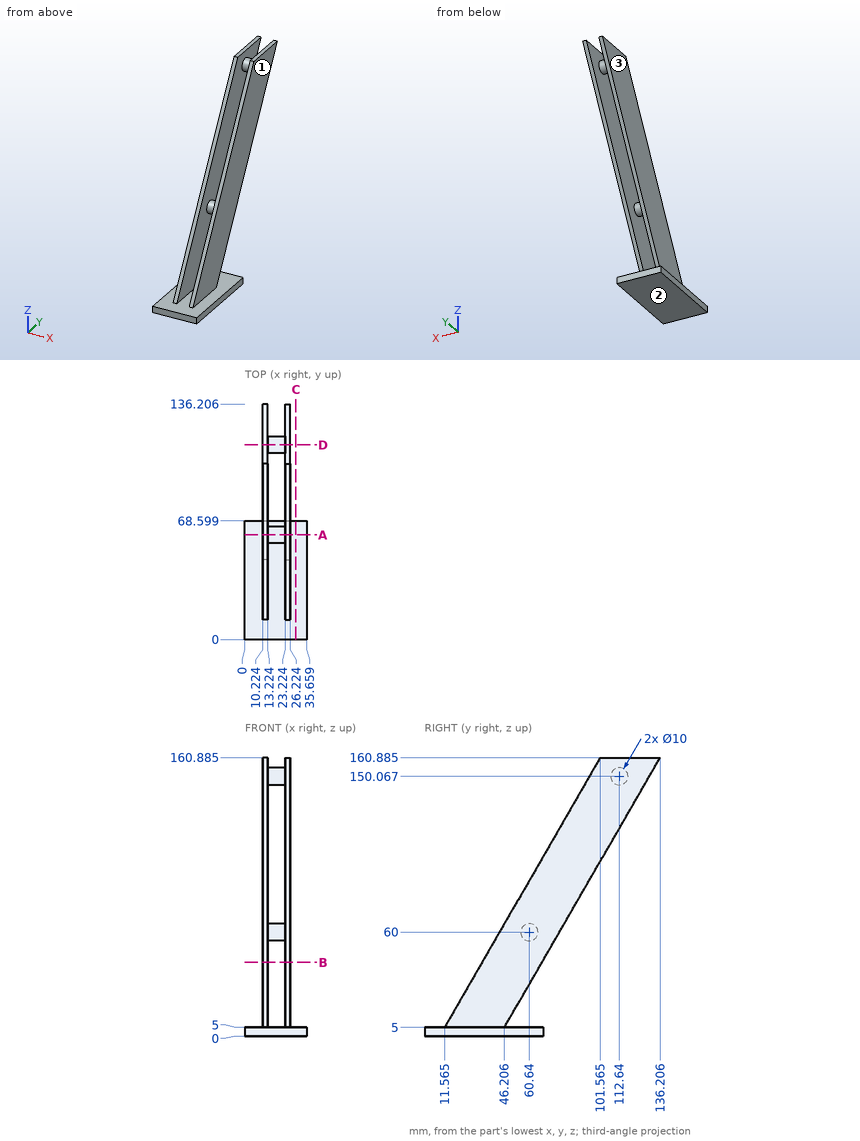
Drawing for the job (mm, zero at the part's lowest x, y, z). A direction names the side the tool comes from. Round coordinates to 2 decimals unless told otherwise and drop trailing zeros. Loops run counter-clockwise (first coordinate to the right, second up) from the corner with the lowest first, then second, coordinate; pieces in that order, holes last. Notation, with made-up numbers: (-39, -32) -> (7, -32) arc R22 ccw to (7, 1) -> close; hole circle Ø3 at (78.5, 53.25). An arc over 180 degrees is marked (long way). Answer as CSV lines item,"result". Start each with the question number.
1) Pin check, flat tips, straight feed: P1, Ø3, axis at x = 16, y = 20, coming from the -Z side; P2, Ø8, axis at x = 9.5, y = 58, coming from the +Z side; P3, Ø1, axis at x = 12.5, z = 138, coming from the +Y side; P4, Ø12, axis at x = 17.5, z = 25, coming from the +Y side. Stop position of each tip, or through.
2) Probe line 1 along X through (y, z) = (70, 65); line 2 along Z through (x, y) = (32, 26); line 3 along Z through (x, y) = (17.5, 58.5). List the from-to ranges inside material, lowest first.
3) Slice it at C-C (x = 29.5). List the corners of the cut face in (y, z), plus the area to 3 significant figures.
4) Slice it at B-B (z = 42.5). List the corners of the cut face in (x, y) (1 decimal), plus the area to 3 significant figures.
5) Slice it at D-D (y = 112.64). List the corners of the cut face in (x, z) (1 decimal), plus the area to 3 significant figures.
6) Tool access for the marked faces 1, 2 and 3: list every direction of +Z, -Z, +X, -X, +Y, -Y with a clear straight run to the whole face (end or side of a thin tool).
7) Slice it at A-A (y = 60.5). List the corners of the cut face in (x, z).
Filled in:
1,P1,"stops at z = 0"
1,P2,"stops at z = 92.24"
1,P3,"stops at y = 123.28"
1,P4,"stops at y = 60.18"
2,line 1,"x = 10.22 to 13.22, 23.22 to 26.22"
2,line 2,"z = 0 to 5"
2,line 3,"z = 0 to 5, 55.48 to 64.52"
3,outline,"(0, 0) -> (68.6, 0) -> (68.6, 5) -> (0, 5) -> close"
3,area,"343 mm2"
4,outline,"(10.2, 33.2) -> (13.2, 33.2) -> (13.2, 67.9) -> (10.2, 67.9) -> close; (23.2, 33.2) -> (26.2, 33.2) -> (26.2, 67.9) -> (23.2, 67.9) -> close"
4,area,"208 mm2"
5,outline,"(10.2, 120.1) -> (13.2, 120.1) -> (13.2, 145.1) -> (23.2, 145.1) -> (23.2, 120.1) -> (26.2, 120.1) -> (26.2, 160.9) -> (23.2, 160.9) -> (23.2, 155.1) -> (13.2, 155.1) -> (13.2, 160.9) -> (10.2, 160.9) -> close"
5,area,"345 mm2"
6,face 1,"+Z, +X, +Y, -Y"
6,face 2,"-Z, +X, -X, +Y, -Y"
6,face 3,"+Z, -X, +Y, -Y"
7,outline,"(0, 0) -> (35.66, 0) -> (35.66, 5) -> (0, 5) -> close; (10.22, 29.76) -> (13.22, 29.76) -> (13.22, 55) -> (23.22, 55) -> (23.22, 29.76) -> (26.22, 29.76) -> (26.22, 89.76) -> (23.22, 89.76) -> (23.22, 65) -> (13.22, 65) -> (13.22, 89.76) -> (10.22, 89.76) -> close"
